```python
from build123d import *

# Parameters (mm, degrees)
SKETCH_1_R      = 1.5
EXTRUDE_1_DEPTH = 1.5
SKETCH_2_W      = 27.94
SKETCH_2_H      = 3
EXTRUDE_2_DEPTH = 10


with BuildPart() as part:
    # Эскиз1 → Бобышка-Вытянуть1 (new body)
    with BuildSketch(Plane(origin=(0, 0, 0), x_dir=(1, 0, 0), z_dir=(0, 1, 0))):
        with BuildLine():
            ThreePointArc((35.56, 22.86), (38.1, 20.32), (35.56, 17.78))
            Line((35.56, 17.78), (33.02, 17.78))
            Line((33.02, 17.78), (33.02, 5.08))
            Line((33.02, 5.08), (35.56, 5.08))
            ThreePointArc((35.56, 5.08), (38.1, 2.54), (35.56, 0))
            Line((35.56, 0), (2.54, 0))
            ThreePointArc((2.54, 0), (0, 2.54), (2.54, 5.08))
            Line((2.54, 5.08), (5.08, 5.08))
            Line((5.08, 5.08), (5.08, 17.78))
            Line((5.08, 17.78), (2.54, 17.78))
            ThreePointArc((2.54, 17.78), (0, 20.32), (2.54, 22.86))
            Line((2.54, 22.86), (35.56, 22.86))
        make_face()
        with Locations(Location((35.56, 2.54, 0), (0, 0, 270))):
            Circle(SKETCH_1_R, mode=Mode.SUBTRACT)
        with Locations(Location((2.54, 2.54, 0), (0, 0, 270))):
            Circle(SKETCH_1_R, mode=Mode.SUBTRACT)
        with Locations(Location((2.54, 20.32, 0), (0, 0, 270))):
            Circle(SKETCH_1_R, mode=Mode.SUBTRACT)
        with Locations(Location((35.56, 20.32, 0), (0, 0, 270))):
            Circle(SKETCH_1_R, mode=Mode.SUBTRACT)
    extrude(amount=EXTRUDE_1_DEPTH)

    # Эскиз2 → Бобышка-Вытянуть2 (add)
    with BuildSketch(Plane(origin=(0, 1.5, 0), x_dir=(1, 0, 0), z_dir=(0, 1, 0))):
        with Locations((19.05, 2.54)):
            Rectangle(SKETCH_2_W, SKETCH_2_H)
    extrude(amount=EXTRUDE_2_DEPTH)


solid = part.part
```
Source: CAD feature listing. Evaluate the final solid. Frame: model axes, mm. A direction names the side the tool comes from. Round coordinates to 2 decimals unless told otherwise and drop trailing zeros. Loops run counter-clockwise (first coordinate to the right, second up) from the corner with the lowest first, then second, coordinate; pieces in that order, holes last. Notation, with made-up numbers: M 73,21 L 77,21 A12 cw 77,35 Z; hole C 69.25,-39 d6. An arc over 180 degrees is marked long. Use a Markdown table: item, result. Add a question column.
1. Section query B-B on x = 4.5. Return the cut outline in (y, z).
2. Line query: line 1 (X direction, y = 0.9, z = -2.54); line 2 (Y direction, x = 5, z = -1.5); line 3 (Z direction, x = 19, y = 6). Output: solid intervals per line, ascending.
3. Contact query for flat-ended pins moving along their axis: P1, Ø3.5, axis at y = 4, z = -2, coming from the -X side; P2, Ø5, axis at x = 14, y = 5.5, coming from the -Z side; P3, Ø7, axis at x = 25, z = -12.5, coming from the +Y side. Output: stop coordinate, or through.
4. Mould query, pull axis X, two halves, no side actions, for faces 5 (the flat face through (4, 1, -5.08)), 6 (the cylindrical face through (38.1, 0.7, -2.6)), 7 (the cylindrical face through (4.027, 0.74, -2.735)), 8 (the cylindrical face through (37.047, 0.74, -2.735)). Classes: pulls with the +X half, pulls with the -X half, needs draft (parallel to the pull), parting line crosses it, or undercut.
5. Section query D-D on z = -2.54. Return the cut outline in (x, y), then the cut area to 3 significant figures.
6. Section query A-A on z = -20.32. Return the cut outline in (x, y), then the cut area to 4 significant figures.
7. Reachability of faces 1 (the flat face through (5.08, 6, -3)), 2 (the flat face through (19, 6, -1.04)), 3 (the flat face through (4, 1, -17.78)), 4 (the flat face through (34, 1, -17.78)) from +Z, -Z, +X, -X, +Y, -Y: full face, straight path, thin tool, end or side. Return the list, or none.
8. Section query C-C on x = 22.5. Return the cut outline in (y, z).
Reported:
| question | item | result |
|---|---|---|
| 1 | outline | M 0,-22.86 L 1.5,-22.86 L 1.5,-17.78 L 0,-17.78 Z; M 0,-5.08 L 1.5,-5.08 L 1.5,0 L 0,0 Z |
| 2 | line 1 | x = 0 to 1.04, 4.04 to 34.06, 37.06 to 38.1 |
| 2 | line 2 | y = 0 to 1.5 |
| 2 | line 3 | z = -4.04 to -1.04 |
| 3 | P1 | stops at x = 5.08 |
| 3 | P2 | stops at z = -4.04 |
| 3 | P3 | stops at y = 1.5 |
| 4 | face 5 | needs draft |
| 4 | face 6 | pulls with the +X half |
| 4 | face 7 | undercut |
| 4 | face 8 | undercut |
| 5 | outline | M 0,0 L 1.04,0 L 1.04,1.5 L 0,1.5 Z; M 4.04,0 L 34.06,0 L 34.06,1.5 L 33.02,1.5 L 33.02,11.5 L 5.08,11.5 L 5.08,1.5 L 4.04,1.5 Z; M 37.06,0 L 38.1,0 L 38.1,1.5 L 37.06,1.5 Z |
| 5 | area | 328 mm² |
| 6 | outline | M 0,0 L 1.04,0 L 1.04,1.5 L 0,1.5 Z; M 4.04,0 L 34.06,0 L 34.06,1.5 L 4.04,1.5 Z; M 37.06,0 L 38.1,0 L 38.1,1.5 L 37.06,1.5 Z |
| 6 | area | 48.15 mm² |
| 7 | face 1 | +Z, -Z, -X, +Y |
| 7 | face 2 | +Z, +X, -X, +Y |
| 7 | face 3 | -X, +Y, -Y |
| 7 | face 4 | +X, +Y, -Y |
| 8 | outline | M 0,-22.86 L 1.5,-22.86 L 1.5,-4.04 L 11.5,-4.04 L 11.5,-1.04 L 1.5,-1.04 L 1.5,0 L 0,0 Z |
